Model file for the job. Use its own axes, mm. Round coordinates to 2 decimals unless told otherwise and drop trailing zeros. Write each loop counter-clockwise with the first axis right and the second up, starting at its lowest first coordinate (ties: lowest second). Pieces come first, ordered by that corner, then holes.
```python
from build123d import *

# Parameters (mm, degrees)
CROQUIS1_W              = 53
CROQUIS1_H              = 7.5
SALIENTE_EXTRUIR1_DEPTH = 9.5
REDONDEO1_RADIUS        = 3.75
REDONDEO1_LENGTH        = 9.5
REDONDEO3_RADIUS        = 3.75
REDONDEO3_LENGTH        = 9.5
CROQUIS2_R              = 1.6
CORTAR_EXTRUIR1_DEPTH   = 29.400044014


with BuildPart() as part:
    # Croquis1 → Saliente-Extruir1 (new body)
    with BuildSketch(Plane(origin=(0, 0, 0), x_dir=(1, 0, 0), z_dir=(0, 1, 0))):
        Rectangle(CROQUIS1_W, CROQUIS1_H)
    extrude(amount=SALIENTE_EXTRUIR1_DEPTH)

    # Redondeo1: full round fillet: the end face becomes a half cylinder, R = half its width
    redondeo1_face = Plane((26.5, 4.75, 0), x_dir=(0, -1, 0), z_dir=(1, 0, 0))  # on the end face: x along it, z out of the body
    redondeo1_slab = redondeo1_face.offset(-REDONDEO1_RADIUS / 2) * Box(REDONDEO1_LENGTH, 2 * REDONDEO1_RADIUS, REDONDEO1_RADIUS, mode=Mode.PRIVATE)  # the body's end, R deep
    redondeo1_round = Plane((22.75, 4.75, 0), x_dir=(1, 0, 0), z_dir=(0, -1, 0)) * Cylinder(REDONDEO1_RADIUS, REDONDEO1_LENGTH, mode=Mode.PRIVATE)  # its axis R under the face
    add(redondeo1_slab - redondeo1_round, mode=Mode.SUBTRACT)

    # Redondeo3: full round fillet: the end face becomes a half cylinder, R = half its width
    redondeo3_face = Plane((-26.5, 4.75, 0), x_dir=(0, 1, 0), z_dir=(-1, 0, 0))  # on the end face: x along it, z out of the body
    redondeo3_slab = redondeo3_face.offset(-REDONDEO3_RADIUS / 2) * Box(REDONDEO3_LENGTH, 2 * REDONDEO3_RADIUS, REDONDEO3_RADIUS, mode=Mode.PRIVATE)  # the body's end, R deep
    redondeo3_round = Plane((-22.75, 4.75, 0), x_dir=(-1, 0, 0), z_dir=(0, 1, 0)) * Cylinder(REDONDEO3_RADIUS, REDONDEO3_LENGTH, mode=Mode.PRIVATE)  # its axis R under the face
    add(redondeo3_slab - redondeo3_round, mode=Mode.SUBTRACT)

    # Croquis2 → Cortar-Extruir1 (cut, through all)
    with BuildSketch(Plane(origin=(0, 9.5, 0), x_dir=(1, 0, 0), z_dir=(0, 1, 0))):
        with Locations(Location((-22.75, 0, 0), (0, 0, 270))):
            Circle(CROQUIS2_R)
        with Locations(Location((22.75, 0, 0), (0, 0, 270))):
            Circle(CROQUIS2_R)
    extrude(amount=-CORTAR_EXTRUIR1_DEPTH, mode=Mode.SUBTRACT)


solid = part.part
```
1) Cut at B-B on y = 2.75. List the corners of the cut face in (x, z).
2) Wall check: probe 1 along X at (y, z) = (5.5, 0); probe 2 along Z at (x, y) = (22, 1.75); probe 3 along X at (y, z) = (3, 3.25). Give the ranges that are in metal, low to high.
3) Pull direction X, two halves, no side cores. Call faces 1 (the face through (0, 5, -3.75)), 2 (the face through (-26.5, 4.8, -0.1)), 3 (the face through (26.5, 4.7, -0.1)), 4 (the face through (-21.164, 4.816, -0.208)): released by +X, released by -X, zero draft, split by the parting line, or undercut.
4) Flat gauge pins, fed straight in: pin 1 Ø2 at (y, z) = (2.5, 1.5) entering from +X; pin 2 Ø1 at (y, z) = (2, 1.5) entering from +X. Where does each tip first touch, or does it go through?
5) Cut at A-A on z = 0. List the corners of the cut face in (x, y).
6) Cut at C-C on z = 2.75. List the corners of the cut face in (x, y).
Result sheet:
1. outline: (-22.75, -3.75) - (22.75, -3.75) arc R3.75 ccw to (22.75, 3.75) - (-22.75, 3.75) arc R3.75 ccw to start; hole circle Ø3.2 at (-22.75, 0); hole circle Ø3.2 at (22.75, 0)
2. probe 1: x = -26.5 to -24.35, -21.15 to 21.15, 24.35 to 26.5
2. probe 2: z = -3.75 to -1.41, 1.41 to 3.75
2. probe 3: x = -24.62 to 24.62
3. face 1: zero draft
3. face 2: released by -X
3. face 3: released by +X
3. face 4: undercut
4. pin 1: stops at x = 26.47
4. pin 2: stops at x = 26.36
5. outline: (-26.5, 0) - (-24.35, 0) - (-24.35, 9.5) - (-26.5, 9.5) - close; (-21.15, 0) - (21.15, 0) - (21.15, 9.5) - (-21.15, 9.5) - close; (24.35, 0) - (26.5, 0) - (26.5, 9.5) - (24.35, 9.5) - close
6. outline: (-25.3, 0) - (25.3, 0) - (25.3, 9.5) - (-25.3, 9.5) - close
